from build123d import *

# Parameters (mm, degrees)
BOSS_EXTRUDE1_DEPTH = 20
BOSS_EXTRUDE2_DEPTH = 140
FILLET1_R           = 10
SKETCH3_R           = 9.999999999999993
CUT_EXTRUDE1_DEPTH  = 282.42494558940575
SKETCH4_R           = 9.999999999999993
CUT_EXTRUDE2_DEPTH  = 279.5677655436824


with BuildPart() as part:
    # Sketch1 → Boss-Extrude1 (new body)
    with BuildSketch(Plane.XY):
        with BuildLine():
            Line((10.000000000000071, 0), (189.99999999999994, 0))
            ThreePointArc((189.99999999999994, 0), (197.07106781186548, 2.92893218813453), (200, 10.000000000000071))
            Line((200, 10.000000000000071), (200, 129.99999999999994))
            ThreePointArc((200, 129.99999999999994), (197.07106781186548, 137.07106781186548), (189.99999999999994, 140))
            Line((189.99999999999994, 140), (10.000000000000071, 140))
            ThreePointArc((10.000000000000071, 140), (2.9289321881345263, 137.07106781186548), (0, 129.99999999999994))
            Line((0, 129.99999999999994), (0, 10.000000000000071))
            ThreePointArc((0, 10.000000000000071), (2.9289321881345254, 2.9289321881345245), (10.000000000000071, 0))
        make_face()
    extrude(amount=-BOSS_EXTRUDE1_DEPTH)

    # Sketch2 → Boss-Extrude2 (add)
    with BuildSketch(Plane(origin=(0, 0, -20), x_dir=(-1, 0, 0), z_dir=(0, 0, -1))):
        Polygon((-180, 140), (-200, 140), (-200, 0), (-179.99999999999997, 2.45e-15), align=None)
    extrude(amount=BOSS_EXTRUDE2_DEPTH)

    # Fillet1
    fillet1_edges = [part.edges().sort_by_distance(p)[0] for p in [
        (190, 1.22e-15, -160),
        (190, 140, -160),
        (180, 70, -20),
        (200, 0, -90),
        (200, 140, -90),
    ]]
    fillet(fillet1_edges, radius=FILLET1_R)

    # Sketch3 → Cut-Extrude1 (cut, through all)
    with BuildSketch(Plane(origin=(0, 0, -20), x_dir=(-1, 0, 0), z_dir=(0, 0, -1))):
        with Locations((-89.99999999999997, 70)):
            Circle(SKETCH3_R)
    extrude(amount=-CUT_EXTRUDE1_DEPTH, mode=Mode.SUBTRACT)

    # Sketch4 → Cut-Extrude2 (cut, through all)
    with BuildSketch(Plane.ZY.offset(-179.99999999999997)):
        with Locations(Location((-90.00000000000001, 70.00000000000003, 0), (0, 0, 270))):
            Circle(SKETCH4_R)
    extrude(amount=-CUT_EXTRUDE2_DEPTH, mode=Mode.SUBTRACT)


solid = part.part
Could you check a few things on this model? Use its own coordinates, in mm. A direction names the side the tool comes from. Give positions to 0.01 mm unless a question says otherwise; leave off trailing zeros. Write each loop counter-clockwise with the first axis right and the second up, starting at its lowest first coordinate (ties: lowest second). Pieces come first, ordered by that corner, then holes. Notation, with made-up numbers: (-27.75, 41.25) -> (31.25, 41.25) arc R11 ccw to (31.25, 50.25) -> close; hole circle Ø10 at (-21, 62). An arc over 180 degrees is marked (long way). Answer as a JSON object with one key per item and string values.
Q1. Will these pins go through, and if not, where does the flat tip stop? pin 1 Ø1.5 at (y, z) = (27.5, -23) entering from -X; pin 2 Ø23 at (x, y) = (90, 70) entering from +Z; pin 3 Ø1 at (x, y) = (127, 86) entering from -Z.
Taken from the geometry:
{"pin 1": "stops at x = 176.32", "pin 2": "stops at z = 0", "pin 3": "stops at z = -20"}
Q2. We'd pull the mould along Y, two halves only. Please class faces 3 (the cylindrical face through (196.99, 2.85, -9.86)), 4 (the flat face through (84, 55, -20)), 5 (the cylindrical face through (189.86, 77.37, -83.24)): released by +Y, released by -Y, zero draft, split by the parting line, or undercut.
Taken from the geometry:
{"face 3": "released by -Y", "face 4": "zero draft", "face 5": "undercut"}
Q3. Suppose I cut it at B-B on z = -90. Write out the boundary of the cut face in (x, y), then the cut area to 3 significant figures.
Taken from the geometry:
{"outline": "(180, 0) -> (190, 0) arc R10 ccw to (200, 10) -> (200, 60) -> (180, 60) -> close; (180, 80) -> (200, 80) -> (200, 130) arc R10 ccw to (190, 140) -> (180, 140) -> close", "area": "2,360 mm²"}
Q4. Suppose I cut it at D-D on y = 30. Write out the boundary of the cut face in (x, z), then the cut area to 3 significant figures.
Taken from the geometry:
{"outline": "(0, -20) -> (170, -20) arc R10 cw to (180, -30) -> (180, -160) -> (200, -160) -> (200, 0) -> (0, 0) -> close", "area": "6,820 mm²"}
Q5. Which directions (+Z, -Z, +X, -X, +Y, -Y) give clear straight access to the entire face, cutting with the end or side of a thin tool? Please do faces 1 (the flat face through (0, 71, -10)), 2 (the flat face through (180, 69, -79.6)).
Taken from the geometry:
{"face 1": "+Z, -Z, -X, +Y, -Y", "face 2": "-Z, -X, +Y, -Y"}
Q6. Please list where these lines run through material, in increasing order: L1, parallel to Z at x = 191, y = 70; L2, parallel to Y at x = 90, z = -7; L3, parallel to Z at x = 80, y = 39.
Taken from the geometry:
{"L1": "z = -160 to -100, -80 to 0", "L2": "y = 0 to 60, 80 to 140", "L3": "z = -20 to 0"}
Q7. Suppose I cut it at C-C on x = 90. Write out the boundary of the cut face in (y, z).
Taken from the geometry:
{"outline": "(0, -20) -> (60, -20) -> (60, 0) -> (0, 0) -> close; (80, -20) -> (140, -20) -> (140, 0) -> (80, 0) -> close"}
Q8. Suppose I cut it at A-A on y = 70. Write out the boundary of the cut face in (x, z).
Taken from the geometry:
{"outline": "(0, -20) -> (80, -20) -> (80, 0) -> (0, 0) -> close; (100, -20) -> (170, -20) arc R10 cw to (180, -30) -> (180, -80) -> (200, -80) -> (200, 0) -> (100, 0) -> close; (180, -160) -> (200, -160) -> (200, -100) -> (180, -100) -> close"}
